Design review of the part shown in the three views and the two pictorial views. Dimensions are in mm from the part's minimum x, y and z. A direction names the side the tool comes from. Round coordinates to 2 decimals unless told otherwise and drop trailing zeros. Write each loop counter-clockwise with the first axis right and the second up, starting at its lowest first coordinate (ties: lowest second). Pieces come first, ordered by that corner, then holes. Notation, with made-up numbers: (6, 20) -> (43, 20) arc R30 cw to (43, 57) -> close; hole circle Ø1 at (-33.75, -2.5). An arc over 180 degrees is marked (long way). Answer as a JSON object with one key per item and string values. Group by question number.
1) To check wall thickness, follow probe 1 along X at (y, z) = (5, 6); probe 2 along Z at (x, y) = (25, 4.85); probe 3 along X at (y, z) = (0.75, 11.25). State the ranges of each line that lie inside material, in increasing order. Write a range as [from, to].
2) We need section D-D, the plane y = 5.5. Write out the cut boundary in (x, z).
3) Mouldability with a two-part tool opening along X and no side actions: class the marked faces 1, 2, 3 and 4 as pulls with the +X half, pulls with the -X half, needs draft (parallel to the pull), parting line crosses it, or undercut.
4) We need section C-C, the plane x = 4.25. Write out the cut boundary in (y, z), then the cut area to 3 significant figures.
5) We need section B-B, the plane z = 6. Write out the cut boundary in (x, y), then the cut area to 3 significant figures.
6) Machinability: for the marked faces 5, 6 and 7, which of the approach directions +Z, -Z, +X, -X, +Y, -Y give a long, thin tool a straight path to every point of the face, cutting with its end or side? Answer none if there is none.
7) Insertion check: pin 1 Ø5.5 at (x, z) = (25, 6) entering from -Y. The pin has a flat end and moves straight along its axis. Give the tip position at first contact, or say it passes through.
8) We need section A-A, the plane y = 1.5. Write out the cut boundary in (x, z).
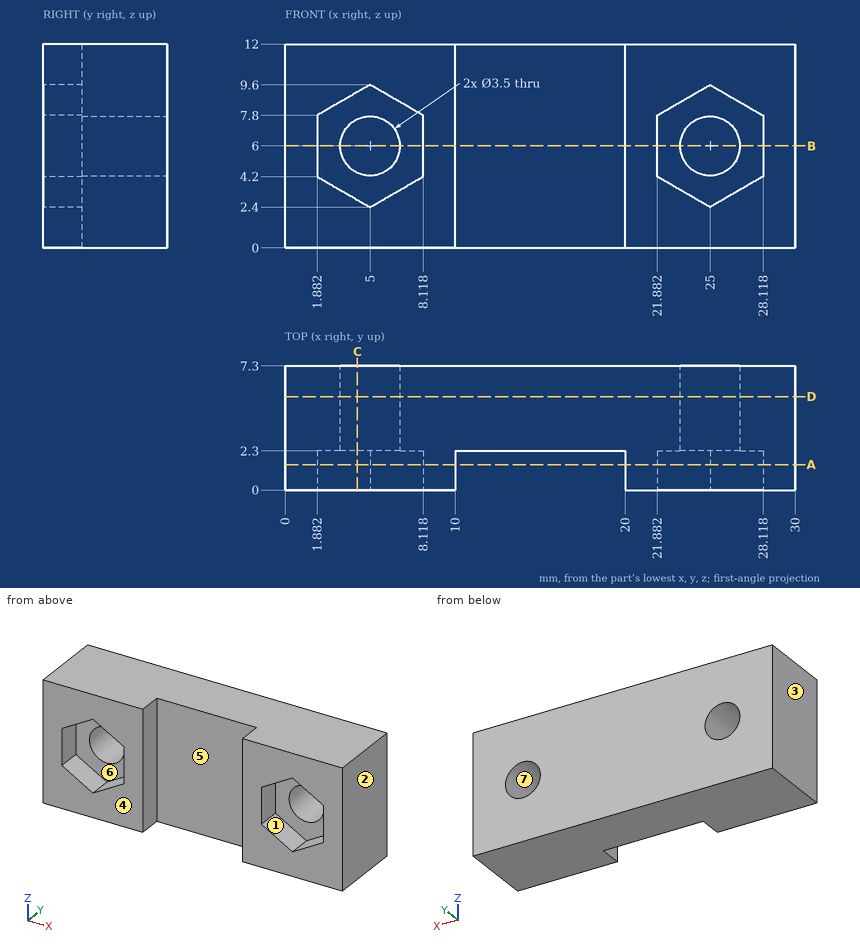
Here are the results:
{
 "1": {"probe 1": "x = [0, 3.25], [6.75, 23.25], [26.75, 30]", "probe 2": "z = [0, 4.25], [7.75, 12]", "probe 3": "x = [0, 10], [20, 30]"},
 "2": {"outline": "(0, 0) -> (30, 0) -> (30, 12) -> (0, 12) -> close; hole circle Ø3.5 at (5, 6); hole circle Ø3.5 at (25, 6)"},
 "3": {"face 1": "undercut", "face 2": "pulls with the +X half", "face 3": "pulls with the -X half", "face 4": "needs draft"},
 "4": {"outline": "(0, 0) -> (7.3, 0) -> (7.3, 4.42) -> (2.3, 4.42) -> (2.3, 2.83) -> (0, 2.83) -> close; (0, 9.17) -> (2.3, 9.17) -> (2.3, 7.58) -> (7.3, 7.58) -> (7.3, 12) -> (0, 12) -> close", "area": "57.2 mm^2"},
 "5": {"outline": "(0, 0) -> (1.88, 0) -> (1.88, 2.3) -> (3.25, 2.3) -> (3.25, 7.3) -> (0, 7.3) -> close; (6.75, 2.3) -> (8.12, 2.3) -> (8.12, 0) -> (10, 0) -> (10, 2.3) -> (20, 2.3) -> (20, 0) -> (21.88, 0) -> (21.88, 2.3) -> (23.25, 2.3) -> (23.25, 7.3) -> (6.75, 7.3) -> close; (26.75, 2.3) -> (28.12, 2.3) -> (28.12, 0) -> (30, 0) -> (30, 7.3) -> (26.75, 7.3) -> close", "area": "132 mm^2"},
 "6": {"face 5": "+Z, -Z, -Y", "face 6": "-Y", "face 7": "+Y, -Y"},
 "7": {"pin 1": "stops at y = 2.3"},
 "8": {"outline": "(0, 0) -> (10, 0) -> (10, 12) -> (0, 12) -> close; (20, 0) -> (30, 0) -> (30, 12) -> (20, 12) -> close; hole (1.88, 4.2) -> (5, 2.4) -> (8.12, 4.2) -> (8.12, 7.8) -> (5, 9.6) -> (1.88, 7.8) -> close; hole (21.88, 4.2) -> (25, 2.4) -> (28.12, 4.2) -> (28.12, 7.8) -> (25, 9.6) -> (21.88, 7.8) -> close"}
}
